Could you check a few things on this model? Use its own coordinates, in mm. Face numbers are marked on the shaded views. A direction names the side the tool comes from. Give positions to 0.01 mm unless a question says otherwise; leave off trailing zeros. Order: outer loops, then holes, each group sorted by start corner. A loop starts at its lowest first (then second) coordinate and runs counter-clockwise, first axis right, second up. Notation, with made-up numbers: M 38,-31.75 L 75,-31.75 A14 ccw 75,-12.75 Z; hole C 30,18.5 d10. An arc over 180 degrees is marked long. Return JSON: item names as keys, results as strings. Group by question number.
```python
from build123d import *

# Parameters (mm, degrees)
F1_DEPTH = 185.42
F3_D     = 6.35
F4_D     = 6.35
F5_D     = 6.35
F6_D     = 6.35
F7_D     = 6.35
F8_D     = 6.35
F9_D     = 6.35
F10_D    = 6.35
F11_D    = 6.35


with BuildPart() as f1:
    # F0 (on Front) → F1 (new body)
    with BuildSketch(Plane.XZ):
        Polygon((84.939852, 17.701955), (-48.410148, 17.701955), (-48.410148, 14.526955), (84.939852, 14.526955), (87.81738, 16.360142), (103.919135, 50.890469), (101.041608, 52.232282), align=None)
    extrude(amount=F1_DEPTH)

    # F3 (through all)
    with Locations(Plane(origin=(62.988826, 0, -29.372172), x_dir=(0, -1, 0), z_dir=(-0.906308, 0, 0.422618))):
        with Locations((18.711276, 77.739262)):
            Hole(F3_D / 2)

    # F4 (through all)
    with Locations(Plane(origin=(62.988826, 0, -29.372172), x_dir=(0, -1, 0), z_dir=(-0.906308, 0, 0.422618))):
        with Locations((12.696845, 69.705941)):
            Hole(F4_D / 2)

    # F5 (through all)
    with Locations(Plane(origin=(62.988826, 0, -29.372172), x_dir=(0, -1, 0), z_dir=(-0.906308, 0, 0.422618))):
        with Locations((19.600639, 62.646478)):
            Hole(F5_D / 2)

    # F6 (through all)
    with Locations(Plane(origin=(62.988826, 0, -29.372172), x_dir=(0, -1, 0), z_dir=(-0.906308, 0, 0.422618))):
        with Locations((25.494844, 69.705941)):
            Hole(F6_D / 2)

    # F7 (through all)
    with Locations(Plane(origin=(62.988826, 0, -29.372172), x_dir=(0, -1, 0), z_dir=(-0.906308, 0, 0.422618))):
        with Locations((166.728864, 77.739262)):
            Hole(F7_D / 2)

    # F8 (through all)
    with Locations(Plane(origin=(62.988826, 0, -29.372172), x_dir=(0, -1, 0), z_dir=(-0.906308, 0, 0.422618))):
        with Locations((160.714432, 69.705987)):
            Hole(F8_D / 2)

    # F9 (through all)
    with Locations(Plane(origin=(62.988826, 0, -29.372172), x_dir=(0, -1, 0), z_dir=(-0.906308, 0, 0.422618))):
        with Locations((167.618226, 62.646478)):
            Hole(F9_D / 2)

    # F10 (through all)
    with Locations(Plane(origin=(62.988826, 0, -29.372172), x_dir=(0, -1, 0), z_dir=(-0.906308, 0, 0.422618))):
        with Locations((173.512431, 69.705987)):
            Hole(F10_D / 2)

    # F11 (through all)
    with Locations(Plane(origin=(62.988826, 0, -29.372172), x_dir=(0, -1, 0), z_dir=(-0.906308, 0, 0.422618))):
        with Locations((93.104638, 69.76501)):
            Hole(F11_D / 2)


solid = f1.part
```
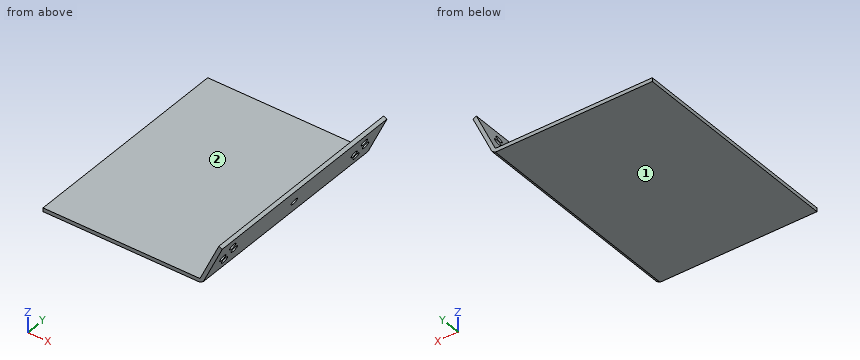
1. Which directions (+Z, -Z, +X, -X, +Y, -Y) give clear straight access to the entire face, cutting with the end or side of a thin tool? Please do the marked faces 1 and 2.
2. Imagine slicing it at B-B, the plane y = -47. Please give me the cut outline in (x, z), plus the area to 3 significant figures.
3. Imagine slicing it at A-A, the plane y = -26. Please give me the cut outline in (x, z).
4. Imagine slicing it at C-C, the plane x = 64.5. Please give me the cut outline in (y, z).
5. For pin 1 (1.5 mm diameter, centred on y = -32, z = 28, fed in from +X); pin 2 (1.5 mm diameter, centred on y = -56, z = 26.5, fed in from -X); pin 3 (10 mm diameter, centred on x = -20.5, y = -153, fed in from +Z), each with a flat end and sliding along its axis, tell me the tip position at first contact or that it passes through.
6. I need wall thicknesses on L1, parallel to Z at x = 7, y = -145.5; L2, parallel to X at y = -159, z = 21.5; L3, parallel to X at y = -53, z = 21. Which ranges of each line are inside material? Lowest first, please. Write a range as from..to.
Values:
{
 "1": {"face 1": "-Z, +X, -X, +Y, -Y", "face 2": "+Z, -X, +Y, -Y"},
 "2": {"outline": "M -48.41,14.53 L 84.94,14.53 L 87.82,16.36 L 103.92,50.89 L 101.04,52.23 L 84.94,17.7 L -48.41,17.7 Z", "area": "549 mm²"},
 "3": {"outline": "M -48.41,14.53 L 84.94,14.53 L 87.82,16.36 L 94,29.62 L 91.12,30.96 L 84.94,17.7 L -48.41,17.7 Z; M 93.77,36.64 L 96.65,35.3 L 103.92,50.89 L 101.04,52.23 Z"},
 "4": {"outline": "M -185.42,14.53 L 0,14.53 L 0,17.7 L -185.42,17.7 Z"},
 "5": {"pin 1": "stops at x = 93.59", "pin 2": "stops at x = 88.69", "pin 3": "stops at z = 17.7"},
 "6": {"L1": "z = 14.53..17.7", "L2": "x = 86.71..90.21", "L3": "x = 86.48..89.98"}
}
